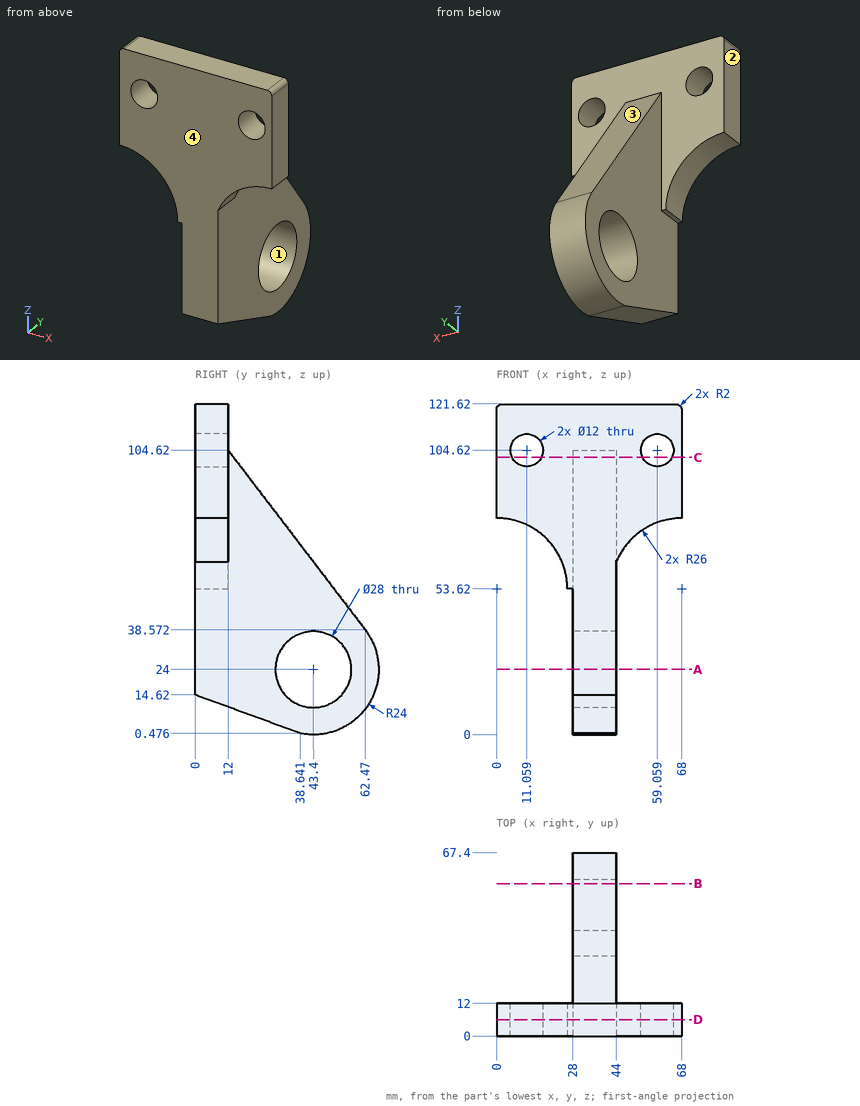
Print and shaded views of the part. All mm, measured from the part's lowest x, y and z. Coordinates: 2 decimals unless noted, no trailing zeros. Write each loop counter-clockwise with the first axis right and the second up, starting at its lowest first coordinate (ties: lowest second). Pieces come first, ordered by that corner, then holes.
(1) Cut at B-B, the plane y = 56. List the corners of the cut face in (x, z).
(2) Cut at A-A, the plane z = 24. List the corners of the cut face in (x, y).
(3) Flat gauge pins, fed straight in: pin 1 (8 mm diameter, centred on y = 9, z = 96, fed in from -X); pin 2 (6 mm diameter, centred on x = 48, y = 17.5, fed in from +Z); pin 3 (20 mm diameter, centred on y = 21, z = 58, fed in from +X); pin 4 (6 mm diameter, centred on x = 23, z = 95, fed in from +Y). Where does each tip first touch, or does it go through?
(4) Two-plate mould, pull along Y, no slides. Class the marked faces 1, 2, 3 and 4: +Y half, -Y half, draft (parallel to the pull), parting line (faces both ways), or undercut.
(5) Cut at D-D, the plane y = 6. List the corners of the cut face in (x, z).
(6) Drill centre lines: probe 1 along Y at (x, z) = (36.5, 24); probe 2 along Y at (x, z) = (16, 81); probe 3 along X at (y, z) = (31, 41). Where is each one in solid material? Low to high.
(7) Cut at C-C, the plane z = 102. List the corners of the cut face in (x, y).
Geometry says:
1. outline: (28, 3.57) - (44, 3.57) - (44, 17.9) - (28, 17.9) - close; (28, 30.1) - (44, 30.1) - (44, 47.04) - (28, 47.04) - close
2. outline: (28, 0) - (44, 0) - (44, 29.4) - (28, 29.4) - close; (28, 57.4) - (44, 57.4) - (44, 67.4) - (28, 67.4) - close
3. pin 1: stops at x = 0
3. pin 2: passes through
3. pin 3: stops at x = 44
3. pin 4: stops at y = 12
4. face 1: undercut
4. face 2: draft
4. face 3: +Y half
4. face 4: -Y half
5. outline: (0, 79.62) arc R26 cw to (26, 53.62) - (28, 53.62) - (28, 12.42) - (44, 12.42) - (44, 63.62) arc R26 cw to (68, 79.62) - (68, 119.62) arc R2 ccw to (66, 121.62) - (2, 121.62) arc R2 ccw to (0, 119.62) - close; hole circle Ø12 at (11.06, 104.62); hole circle Ø12 at (59.06, 104.62)
6. probe 1: y = 0 to 29.4, 57.4 to 67.4
6. probe 2: y = 0 to 12
6. probe 3: x = 28 to 44
7. outline: (0, 0) - (5.66, 0) - (5.66, 12) - (0, 12) - close; (16.46, 0) - (53.66, 0) - (53.66, 12) - (44, 12) - (44, 14) - (28, 14) - (28, 12) - (16.46, 12) - close; (64.46, 0) - (68, 0) - (68, 12) - (64.46, 12) - close
